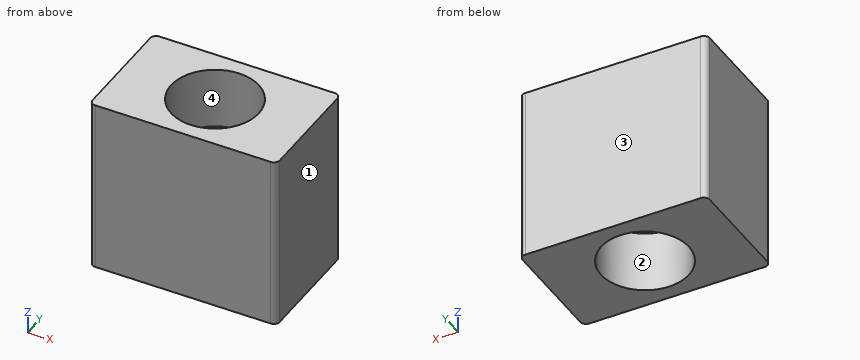
```python
from build123d import *

# Parameters (mm, degrees)
SKETCH1_R           = 5.25
BOSS_EXTRUDE1_DEPTH = 15
SKETCH2_R           = 7.5
CUT_EXTRUDE1_DEPTH  = 10.5


with BuildPart() as part:
    # Sketch1 → Boss-Extrude1 (new, symmetric)
    with BuildSketch(Plane.XY):
        with BuildLine():
            Line((-15, 10), (15, 10))
            ThreePointArc((15, 10), (15.707106781, 9.707106781), (16, 9))
            Line((16, 9), (16, -9))
            ThreePointArc((16, -9), (15.707106781, -9.707106781), (15, -10))
            Line((15, -10), (-15, -10))
            ThreePointArc((-15, -10), (-15.707106781, -9.707106781), (-16, -9))
            Line((-16, -9), (-16, 9))
            ThreePointArc((-16, 9), (-15.707106781, 9.707106781), (-15, 10))
        make_face()
        Circle(SKETCH1_R, mode=Mode.SUBTRACT)
    extrude(amount=BOSS_EXTRUDE1_DEPTH, both=True)

    # Sketch2 → Cut-Extrude1 (cut)
    with BuildSketch(Plane.XY.offset(15)):
        Circle(SKETCH2_R)
    cut_extrude1 = extrude(amount=-CUT_EXTRUDE1_DEPTH, mode=Mode.SUBTRACT)

    # Mirror1: Cut-Extrude1 across plane
    add(cut_extrude1.mirror(Plane.XY), mode=Mode.SUBTRACT)


solid = part.part
```
Geometry: final body of the model. Coordinates: model frame, mm. Face numbers are marked on the shaded views. Coordinates: 2 decimals unless noted, no trailing zeros. Loops run counter-clockwise (first coordinate to the right, second up) from the corner with the lowest first, then second, coordinate; pieces in that order, holes last. Notation, with made-up numbers: (73.25, 26) -> (90.25, 26) arc R27 ccw to (90.25, 63) -> close; hole circle Ø10 at (55, 69.5). An arc over 180 degrees is marked (long way). Use a Markdown table: item, result. Add a question column.
(1) Mould query, pull axis X, two halves, no side actions, for the marked faces 1, 2, 3 and 4. Classes: pulls with the +X half, pulls with the -X half, needs draft (parallel to the pull), parting line crosses it, or undercut.
(2) Line query: line 1 along X through (y, z) = (0.25, -9.25); line 2 along X through (y, z) = (0, -1.5); line 3 along Y through (x, z) = (0, 1.5). Output: solid intervals per line, ascending.
(3) Section query B-B, the plane x = 0. Return loops of the section in (y, z).
(4) Section query D-D, the plane y = 6. Return loops of the section in (x, z), plus the area to 3 significant figures.
(5) Pin query (flat end, axial travel): pin 1 Ø9.5 at (x, y) = (0, 0) entering from +Z; pin 2 Ø7.5 at (x, y) = (-2.5, -2.5) entering from -Z. Return the tip coordinate at first contact, or that it passes through.
(6) Section query A-A, the plane y = 0. Return loops of the section in (x, z).
(7) Section query C-C, the plane z = -2.5. Return loops of the section in (x, y), plus the area to 3 significant figures.
Answer:
| question | item | result |
|---|---|---|
| 1 | face 1 | pulls with the +X half |
| 1 | face 2 | undercut |
| 1 | face 3 | needs draft |
| 1 | face 4 | undercut |
| 2 | line 1 | x = -16 to -7.5, 7.5 to 16 |
| 2 | line 2 | x = -16 to -5.25, 5.25 to 16 |
| 2 | line 3 | y = -10 to -5.25, 5.25 to 10 |
| 3 | outline | (-10, -15) -> (-7.5, -15) -> (-7.5, -4.5) -> (-5.25, -4.5) -> (-5.25, 4.5) -> (-7.5, 4.5) -> (-7.5, 15) -> (-10, 15) -> close; (5.25, -4.5) -> (7.5, -4.5) -> (7.5, -15) -> (10, -15) -> (10, 15) -> (7.5, 15) -> (7.5, 4.5) -> (5.25, 4.5) -> close |
| 4 | outline | (-16, -15) -> (-4.5, -15) -> (-4.5, -4.5) -> (4.5, -4.5) -> (4.5, -15) -> (16, -15) -> (16, 15) -> (4.5, 15) -> (4.5, 4.5) -> (-4.5, 4.5) -> (-4.5, 15) -> (-16, 15) -> close |
| 4 | area | 771 mm^2 |
| 5 | pin 1 | passes through |
| 5 | pin 2 | stops at z = -4.5 |
| 6 | outline | (-16, -15) -> (-7.5, -15) -> (-7.5, -4.5) -> (-5.25, -4.5) -> (-5.25, 4.5) -> (-7.5, 4.5) -> (-7.5, 15) -> (-16, 15) -> close; (5.25, -4.5) -> (7.5, -4.5) -> (7.5, -15) -> (16, -15) -> (16, 15) -> (7.5, 15) -> (7.5, 4.5) -> (5.25, 4.5) -> close |
| 7 | outline | (-16, -9) arc R1 ccw to (-15, -10) -> (15, -10) arc R1 ccw to (16, -9) -> (16, 9) arc R1 ccw to (15, 10) -> (-15, 10) arc R1 ccw to (-16, 9) -> close; hole circle Ø10.5 at (0, 0) |
| 7 | area | 553 mm^2 |
